Input: part model. Units: mm. Frame: model coordinates. A direction names the side the tool comes from. Round coordinates to 2 decimals unless told otherwise and drop trailing zeros. Loops run counter-clockwise (first coordinate to the right, second up) from the corner with the lowest first, then second, coordinate; pieces in that order, holes last. Notation, with made-up numbers: (88, 81.5) -> (100, 81.5) arc R30 ccw to (100, 110.5) -> close; hole circle Ø5 at (67, -4.75). An arc over 180 degrees is marked (long way). Answer in a Markdown table with one row per item. Add a question column.
Q1. Ray query, L1, parallel to X at y = -8.6, z = 7.25; L2, parallel to X at y = -5, z = 7.25; L3, parallel to Y at x = 13.25, z = 5. Return the intervals inside material, ascending. Write a range as from..to.
Q2. Mould query, pull axis X, two halves, no side actions, for faces 1 (the face through (30.854, -7, 7)), 2 (the face through (28.44, -6.27, 8.77)), 3 (the face through (4, 1, 0)). Classes: pulls with the +X half, pulls with the -X half, needs draft (parallel to the pull), parting line crosses it, or undercut.
Q3. Reachability of faces 4 (the face through (13.2, 15, 0.6)), 5 (the face through (28.464, -6.271, 5.771)), 6 (the face through (2.19, -4.82, 6.83)), 7 (the face through (16, 7, 7)) from +Z, -Z, +X, -X, +Y, -Y: full face, straight path, thin tool, end or side. Return the list, or none.
Q4. Section B-B, the plane z = 2.25. Output: boundary loops of the cut face in (x, y).
Q5. Section C-C, the plane x = 13.25. Output: boundary loops of the cut face in (y, z).
Q6. Section A-A, the plane y = -6.5. Output: boundary loops of the cut face in (x, z).
Q7. Section D-D, the plane y = 17.5. Output: boundary loops of the cut face in (x, z), and give its area (3 significant figures).
Q8. Pin query (flat end, axial travel): pin 1 (12 mm diameter, centred on x = 15.5, y = -3.5, fed in from -Z); pin 2 (2.5 mm diameter, centred on x = 2.75, y = 2.5, fed in from -Z); pin 3 (3 mm diameter, centred on y = 13.5, z = 4.5, fed in from +X); pin 4 (2 mm diameter, centred on x = 0.85, z = 7.25, fed in from -Y). Return the tip coordinate at first contact, or that it passes through.
```python
from build123d import *

# Parameters (mm, degrees)
SKETCH1_R             = 2.5
SKETCH1_R_2           = 1.5
BOSS_EXTRUDE1_DEPTH   = 1.25
BOSS_EXTRUDE1_2_DEPTH = 1.25
BOSS_EXTRUDE1_3_DEPTH = 1.25
BOSS_EXTRUDE2_START   = 1.25
SKETCH1_3_W           = 16
SKETCH1_3_H           = 29.4
SKETCH1_3_R           = 2.5
SKETCH1_3_R_2         = 1.5
BOSS_EXTRUDE2_DEPTH   = 12
SKETCH2_W             = 35.854037965
SKETCH2_H             = 12
BOSS_EXTRUDE3_DEPTH   = 5
SKETCH2_3_W           = 35.854037965
SKETCH2_3_H           = 11
SKETCH2_3_R           = 1.75
SKETCH2_3_R_2         = 1.4
BOSS_EXTRUDE4_DEPTH   = 3
SKETCH2_4_R           = 1.4
CUT_EXTRUDE1_DEPTH    = 10
SKETCH2_5_R           = 1.75
BOSS_EXTRUDE5_DEPTH   = 2


with BuildPart() as part:
    # Sketch1 → Boss-Extrude1 (new body)
    with BuildSketch(Plane.XY):
        with Locations((2.75, 17.5)):
            Circle(SKETCH1_R)
        with Locations((2.75, 17.5)):
            Circle(SKETCH1_R_2, mode=Mode.SUBTRACT)
    extrude(amount=BOSS_EXTRUDE1_DEPTH)



with BuildPart() as body_2:
    # Sketch1 → Boss-Extrude1 2 (new body)
    with BuildSketch(Plane.XY):
        with BuildLine():
            Line((14.339724736, 19.75), (12.160275264, 19.75))
            ThreePointArc((12.160275264, 19.75), (13.25, 15), (14.339724736, 19.75))
        make_face()
        with Locations((13.25, 17.5)):
            Circle(SKETCH1_R_2, mode=Mode.SUBTRACT)
    extrude(amount=BOSS_EXTRUDE1_2_DEPTH)


with BuildPart() as body_3:
    # Sketch1 → Boss-Extrude1 3 (new body)
    with BuildSketch(Plane.XY):
        with Locations((2.75, 2.5)):
            Circle(SKETCH1_R)
        with Locations((2.75, 2.5)):
            Circle(SKETCH1_R_2, mode=Mode.SUBTRACT)
    extrude(amount=BOSS_EXTRUDE1_3_DEPTH)


with BuildPart() as part_1:
    add(part.part)

    add(body_2.part)  # Boss-Extrude2 merges body 2

    add(body_3.part)  # Boss-Extrude2 merges body 3
    # Sketch1<3> → Boss-Extrude2 (add)
    with BuildSketch(Plane.XY.offset(BOSS_EXTRUDE2_START)):
        with Locations((8, 5.05)):
            Rectangle(SKETCH1_3_W, SKETCH1_3_H)
        with Locations((13.25, 17.5)):
            Circle(SKETCH1_3_R, mode=Mode.SUBTRACT)
        with Locations((2.75, 17.5)):
            Circle(SKETCH1_3_R, mode=Mode.SUBTRACT)
        with Locations((2.75, 2.5)):
            Circle(SKETCH1_3_R, mode=Mode.SUBTRACT)
        with Locations((2.75, 2.5)):
            Circle(SKETCH1_3_R)
        with Locations((2.75, 2.5)):
            Circle(SKETCH1_3_R_2, mode=Mode.SUBTRACT)
        with BuildLine():
            Line((3.839724736, 19.75), (1.660275264, 19.75))
            ThreePointArc((1.660275264, 19.75), (1.422278614, 15.381709198), (5.25, 17.5))
            ThreePointArc((5.25, 17.5), (4.868290802, 18.827721386), (3.839724736, 19.75))
        make_face()
        with Locations((2.75, 17.5)):
            Circle(SKETCH1_3_R_2, mode=Mode.SUBTRACT)
        with BuildLine():
            Line((14.339724736, 19.75), (12.160275264, 19.75))
            ThreePointArc((12.160275264, 19.75), (11.922278614, 15.381709198), (15.75, 17.5))
            ThreePointArc((15.75, 17.5), (15.368290802, 18.827721386), (14.339724736, 19.75))
        make_face()
        with Locations((13.25, 17.5)):
            Circle(SKETCH1_3_R_2, mode=Mode.SUBTRACT)
    extrude(amount=BOSS_EXTRUDE2_DEPTH)

    # Sketch2 → Boss-Extrude3 (add)
    with BuildSketch(Plane(origin=(0, -9.75, 0), x_dir=(1, 0, 0), z_dir=(0, 1, 0))):
        with Locations((12.927018983, -7.25)):
            Rectangle(SKETCH2_W, SKETCH2_H)
        Polygon((29.31813958, -7.25), (27.586088773, -4.25), (24.121987157, -4.25), (22.38993635, -7.25), (24.121987157, -10.25), (27.586088773, -10.25), align=None, mode=Mode.SUBTRACT)
    extrude(amount=BOSS_EXTRUDE3_DEPTH)

    # Sketch2<3> → Boss-Extrude4 (add)
    with BuildSketch(Plane(origin=(0, -9.75, 0), x_dir=(1, 0, 0), z_dir=(0, 1, 0))):
        with Locations((12.927018983, -7.25)):
            Rectangle(SKETCH2_3_W, SKETCH2_3_H)
        with Locations((0.854037965, -7.25)):
            Circle(SKETCH2_3_R, mode=Mode.SUBTRACT)
        Polygon((27.586088773, -4.25), (29.31813958, -7.25), (27.586088773, -10.25), (24.121987157, -10.25), (22.38993635, -7.25), (24.121987157, -4.25), align=None, mode=Mode.SUBTRACT)
        with Locations((0.854037965, -7.25)):
            Circle(SKETCH2_3_R_2)
    extrude(amount=BOSS_EXTRUDE4_DEPTH)

    # Sketch2<4> → Cut-Extrude1 (cut)
    with BuildSketch(Plane(origin=(0, -9.75, 0), x_dir=(1, 0, 0), z_dir=(0, 1, 0))):
        with Locations((0.854037965, -7.25)):
            Circle(SKETCH2_4_R)
    extrude(amount=CUT_EXTRUDE1_DEPTH, mode=Mode.SUBTRACT)

    # Sketch2<5> → Boss-Extrude5 (add)
    with BuildSketch(Plane(origin=(0, -9.75, 0), x_dir=(1, 0, 0), z_dir=(0, 1, 0))):
        Polygon((24.121987157, -10.25), (27.586088773, -10.25), (29.31813958, -7.25), (27.586088773, -4.25), (24.121987157, -4.25), (22.38993635, -7.25), align=None)
        with Locations((25.854037965, -7.25)):
            Circle(SKETCH2_5_R, mode=Mode.SUBTRACT)
    extrude(amount=BOSS_EXTRUDE5_DEPTH)


solid = part_1.part
```
Answer block:
| question | item | result |
|---|---|---|
| 1 | L1 | -5..-0.55, 2.25..24.1, 27.6..30.85 |
| 1 | L2 | -5..-0.55, 2.25..22.39, 29.32..30.85 |
| 1 | L3 | -9.75..16, 19..19.75 |
| 2 | face 1 | pulls with the +X half |
| 2 | face 2 | undercut |
| 2 | face 3 | needs draft |
| 3 | face 4 | -Z |
| 3 | face 5 | +Y |
| 3 | face 6 | -Y |
| 3 | face 7 | +Z, -Z, +X, +Y |
| 4 | outline | (-5, -9.75) -> (30.85, -9.75) -> (30.85, -4.75) -> (16, -4.75) -> (16, 19.75) -> (0, 19.75) -> (0, -4.75) -> (-5, -4.75) -> close; hole circle Ø3 at (2.75, 2.5); hole circle Ø3 at (2.75, 17.5); hole circle Ø3 at (13.25, 17.5) |
| 5 | outline | (-9.75, 1.25) -> (15, 1.25) -> (15, 0) -> (16, 0) -> (16, 13.25) -> (-9.75, 13.25) -> close; (19, 0) -> (19.75, 0) -> (19.75, 13.25) -> (19, 13.25) -> close |
| 6 | outline | (-5, 1.25) -> (30.85, 1.25) -> (30.85, 13.25) -> (-5, 13.25) -> close; hole circle Ø2.8 at (0.85, 7.25); hole (22.39, 7.25) -> (24.12, 4.25) -> (27.59, 4.25) -> (29.32, 7.25) -> (27.59, 10.25) -> (24.12, 10.25) -> close |
| 7 | outline | (0, 1.25) -> (0.25, 1.25) -> (0.25, 0) -> (1.25, 0) -> (1.25, 13.25) -> (0, 13.25) -> close; (4.25, 0) -> (5.25, 0) -> (5.25, 1.25) -> (10.75, 1.25) -> (10.75, 0) -> (11.75, 0) -> (11.75, 13.25) -> (4.25, 13.25) -> close; (14.75, 0) -> (15.75, 0) -> (15.75, 1.25) -> (16, 1.25) -> (16, 13.25) -> (14.75, 13.25) -> close |
| 7 | area | 125 mm^2 |
| 8 | pin 1 | z = 1.25 |
| 8 | pin 2 | through |
| 8 | pin 3 | x = 16 |
| 8 | pin 4 | y = 0.25 |
